Here's how the part is built. I have some questions about the finished solid (model axes, mm). Round coordinates to 2 decimals unless told otherwise and drop trailing zeros. Order: outer loops, then holes, each group sorted by start corner. A loop starts at its lowest first (then second) coordinate and runs counter-clockwise, first axis right, second up.
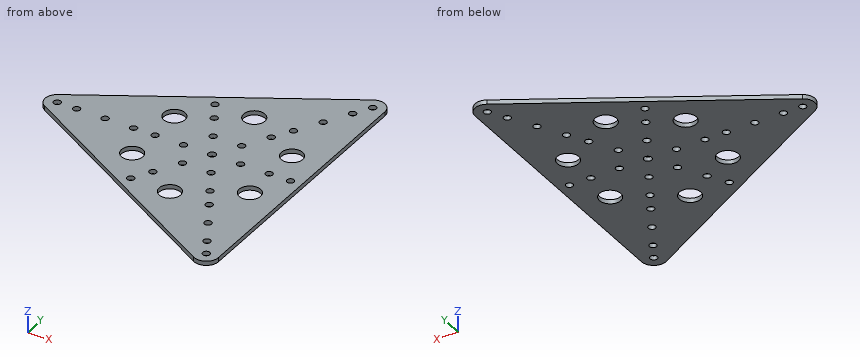
Autodesk Inventor part; units mm, degrees
ref_plane "YZ Plane" through (0, 0, 0) normal (1, 0, 0) x (0, 1, 0)
ref_plane "XZ Plane" through (0, 0, 0) normal (0, 1, 0) x (-1, 0, 0)
ref_plane "XY Plane" through (0, 0, 0) normal (0, 0, 1) x (1, 0, 0)
sketch "Sketch1" plane through (0, 0, 0) normal (0, 0, 1) x (1, 0, 0)
  line L0 (-154.4076, 199.4033) -> (65.098, -180.7915)
  circle A0 centre (-39.282, 0) radius 2.75
  circle A1 centre (15, 94.0192) radius 8.5
  circle A2 centre (-147.8461, 0) radius 8.5
  circle A3 centre (15, -94.0192) radius 8.5
  line L1 (15, 94.0192) -> (15, -94.0192)
  line L2 (15, -94.0192) -> (-147.8461, 0)
  line L3 (-147.8461, 0) -> (15, 94.0192)
  line L4 (53.7758, 126.2214) -> (-193.87, -16.757)
  line L5 (23.5, -175.7783) -> (23.5, 120.7175)
  line L6 (64.2969, -132.2958) -> (-207.0406, 24.361)
  circle A4 centre (-39.282, 0) radius 2.75
  circle A5 centre (-39.282, 0) radius 2.5
  point P0 (0, 0)
  point P1 (23.5, -94.0192)
  point P2 (23.5, 94.0192)
  point P3 (10.75, 101.3805)
  point P4 (-152.0961, 7.3612)
  point P5 (-152.0961, -7.3612)
  point P6 (10.75, -101.3805)
  dimension "d2" = 17
  dimension "d3" = 360
  dimension "d4" = 5.5
extrude "Extrusion1" add sketch "Sketch1" along normal blind 3 contours L4 A1 L3 L0 | L0 L3 A2 L4 | L3 A1 L1 A3 L0 A0 | L0 A0 A3 L2 A2 L3 | A1 L1 L3 | A2 L3 L2 | A2 L2 L3 | L3 L1 A1 | L5 A3 L1 A1 | A2 L2 A3 L6 | A3 L0 L1 | A3 L2 L0 | A3 L1 L0 | L0 L2 A3
sketch "Sketch2" plane through (0, 0, 3) normal (0, 0, 1) x (1, 0, 0)
  circle A0 centre (-147.8461, 0) radius 2.5
  circle A1 centre (15, 94.0192) radius 2.5
  circle A2 centre (15, -94.0192) radius 2.5
  line L0 (-152.0961, -7.3612) -> (10.75, -101.3805)
  line L1 (10.75, 101.3805) -> (-152.0961, 7.3612)
  point P0 (0, 0)
extrude "Extrusion2" cut sketch "Sketch2" against normal blind 3
sketch "Sketch3" plane through (0, 0, 3) normal (0, 0, 1) x (1, 0, 0)
  circle A0 centre (-39.282, 0) radius 2.75
  line L0 (-39.282, 0) -> (-59.282, 0)
  line L1 (-59.282, 0) -> (-79.282, 0)
  line L2 (-79.282, 0) -> (-94.282, 0)
  line L3 (-94.282, 0) -> (-109.282, 0)
  line L4 (-59.282, 0) -> (-49.282, 17.3205)
  line L5 (-49.282, 17.3205) -> (-29.282, 17.3205)
  line L6 (-29.282, 17.3205) -> (-19.282, 0)
  line L7 (-19.282, 0) -> (-29.282, -17.3205)
  line L8 (-29.282, -17.3205) -> (-49.282, -17.3205)
  line L9 (-49.282, -17.3205) -> (-59.282, 0)
  line L10 (-79.282, 0) -> (-59.282, 34.641)
  line L11 (-59.282, 34.641) -> (-19.282, 34.641)
  line L12 (-19.282, 34.641) -> (0.718, 0)
  line L13 (0.718, 0) -> (-19.282, -34.641)
  line L14 (-19.282, -34.641) -> (-59.282, -34.641)
  line L15 (-59.282, -34.641) -> (-79.282, 0)
  line L16 (-94.282, 0) -> (-66.782, 47.6314)
  line L17 (-66.782, 47.6314) -> (-11.782, 47.6314)
  line L18 (-11.782, 47.6314) -> (15.718, 0)
  line L19 (15.718, 0) -> (-11.782, -47.6314)
  line L20 (-11.782, -47.6314) -> (-66.782, -47.6314)
  line L21 (-66.782, -47.6314) -> (-94.282, 0)
  circle A1 centre (-49.282, -17.3205) radius 2.5
  circle A2 centre (-59.282, -34.641) radius 2.5
  circle A3 centre (-66.782, -47.6314) radius 2.5
  circle A4 centre (-29.282, -17.3205) radius 2.5
  circle A5 centre (-19.282, -34.641) radius 2.5
  circle A6 centre (-11.782, -47.6314) radius 2.5
  circle A7 centre (-19.282, 0) radius 2.5
  circle A8 centre (0.718, 0) radius 2.5
  circle A9 centre (15.718, 0) radius 2.5
  circle A10 centre (-29.282, 17.3205) radius 2.5
  circle A11 centre (-19.282, 34.641) radius 2.5
  circle A12 centre (-11.782, 47.6314) radius 2.5
  circle A13 centre (-49.282, 17.3205) radius 2.5
  circle A14 centre (-59.282, 34.641) radius 2.5
  circle A15 centre (-66.782, 47.6314) radius 2.5
  circle A16 centre (-59.282, 0) radius 2.5
  circle A17 centre (-79.282, 0) radius 2.5
  circle A18 centre (-94.282, 0) radius 2.5
  line L22 (-19.282, -34.641) -> (-11.782, -47.6314)
  line L23 (-11.782, -47.6314) -> (-1.782, -64.9519)
  line L24 (-1.782, -64.9519) -> (8.218, -82.2724)
  circle A19 centre (-1.782, -64.9519) radius 2.5
  circle A20 centre (8.218, -82.2724) radius 2.5
  circle A21 centre (-1.782, 64.9519) radius 2.5
  circle A22 centre (8.218, 82.2724) radius 2.5
  circle A23 centre (-114.282, 0) radius 2.5
  circle A24 centre (-134.282, 0) radius 2.5
  line L25 (-80.532, 23.8157) -> (-39.282, 0)
  line L26 (-39.282, 0) -> (-39.282, 47.6314)
  line L27 (-39.282, 0) -> (1.968, 23.8157)
  line L28 (-39.282, 0) -> (1.968, -23.8157)
  line L29 (-39.282, 0) -> (-39.282, -47.6314)
  line L30 (-39.282, 0) -> (-80.532, -23.8157)
  circle A25 centre (-80.532, -23.8157) radius 7.5
  circle A26 centre (-39.282, -47.6314) radius 7.5
  circle A27 centre (1.968, -23.8157) radius 7.5
  circle A28 centre (1.968, 23.8157) radius 7.5
  circle A29 centre (-39.282, 47.6314) radius 7.5
  circle A30 centre (-80.532, 23.8157) radius 7.5
  point P0 (0, 0)
  dimension "d9" = 20
  dimension "d10" = 20
  dimension "d11" = 15
  dimension "d12" = 15
  dimension "d13" = 5
  dimension "d14" = 5
  dimension "d15" = 5
  dimension "d18" = 360
  dimension "d20" = 20
  dimension "d21" = 20
  dimension "d22" = 5
  dimension "d23" = 5
  dimension "d24" = 17.3205
  dimension "d27" = 360
  dimension "d31" = 15
  dimension "d32" = 15
  dimension "d33" = 15
  dimension "d34" = 15
  dimension "d35" = 15
  dimension "d36" = 15
extrude "Extrusion3" cut sketch "Sketch3" against normal blind 3 contours A10 L5 L6 | L6 L5 A10 | A7 L7 L6 | L6 L7 A7 | A4 L8 L7 | L7 L8 A4 | A13 L4 L5 | L5 L4 A13 | A16 L9 L0 | L0 L4 A16 | A11 L11 L12 | L12 L11 A11 | A8 L13 L12 | L12 L13 A8 | A28 L18 L27 | L27 L18 A28 | A1 L9 L8 | L8 L9 A1 | A5 L22 L13 | L13 L14 A5 | A27 L19 L28 | L28 L19 A27 | L4 L1 A16 | A14 L10 L11 | L11 L10 A14 | A29 L17 L26 | L26 L17 A29 | L9 A16 L1 | L18 A28 | A20 | A19 L24 L23 | L23 L24 A19 | L14 L22 A5 | A2 L15 L14 | L14 L15 A2 | A26 L20 L29 | L29 L20 A26 | L19 A27 | A17 L1 L10 | L10 L2 A17 | A30 L16 L25 | L25 L16 A30 | L17 A29 | A17 L2 L15 | L15 L1 A17 | A25 L21 L30 | L30 L21 A25 | A12 L17 L18 | L18 L17 A12 | A9 L19 L18 | L18 L19 A9 | L20 A26 | A6 L23 L19 | L19 L22 A6 | L16 A30 | A15 L16 L17 | L17 L16 A15 | L21 A25 | L22 L20 A6 | L20 L23 A6 | A3 L21 L20 | L20 L21 A3 | A18 L21 L2 | L2 L16 A18 | L16 L3 A18 | A18 L3 L21 | A21 | A22 | A23 | A24
properties part number "multifunctional_lvl"
1) If we section it at A-A (y = 0): Give the number of separate pieces and of enclosed holes in the cut face, plus the area to 3 significant figures.
2) If we section it at C-C (x = -100): Write out the boundary of the cut face in (y, z).
3) I'm going to push flat-ended pins straight in: pin 1 (1.5 mm diameter, centred on x = -84, z = 1.5, fed in from -Y); pin 2 (1 mm diameter, centred on x = -52.5, z = 1.5, fed in from -Y); pin 3 (1 mm diameter, centred on y = -30.5, z = 1.5, fed in from -X). Where does each tip first touch, or does it pass through?
4) I need wall thicknesses on line 1 (Y direction, x = -18.5, z = 1.8); line 2 (X direction, y = 48, z = 1.15); line 3 (X direction, y = 20.5, z = 1.3). Which ranges of each line are inside material? Lowest first, please.
5) If we section it at D-D (y = 76.5): Write out the boundary of the cut face in (x, z).
Solutions:
1. separate pieces: 11
1. enclosed holes: 0
1. area: 388 mm2
2. outline: (-37.44, 0) - (37.44, 0) - (37.44, 3) - (-37.44, 3) - close
3. pin 1: stops at y = -47.11
3. pin 2: stops at y = -65.15
3. pin 3: stops at x = -112.88
4. line 1: y = -84.49 to -37.02, -32.27 to -2.37, 2.37 to 32.27, 37.02 to 84.49
4. line 2: x = -81.71 to -69.25, -64.31 to -46.77, -31.79 to -14.25, -9.31 to 23.5
4. line 3: x = -129.34 to -87.26, -73.8 to -4.76, 8.7 to 23.5
5. outline: (-32.34, 0) - (23.5, 0) - (23.5, 3) - (-32.34, 3) - close
